The listing builds one solid part. Answer for the finished solid, in the listing's coordinates (mm). Give positions to 0.01 mm unless a question says otherwise; leave off trailing zeros. Order: outer loops, then holes, each group sorted by start corner. A loop starts at its lowest first (then second) coordinate and runs counter-clockwise, first axis right, second up. Notation, with made-up numbers: (-5, -39) - (14, -39) arc R16 ccw to (14, -34) - close; hole circle Ø6 at (-11, 81.5). An arc over 180 degrees is marked (long way). Answer in a Markdown table with one row per item. Add a question column.
```python
from build123d import *

# Parameters (mm, degrees)
F0_W          = 70
F0_H          = 70
F0_W_2        = 1860
F0_H_2        = 360
F1_DEPTH      = 70
F2_W          = 360
F2_H          = 30
F3_DEPTH      = 25
F3_DEPTH_BACK = 25
F4_SCALE      = 0.4


with BuildPart() as f1:
    # F0 (on Front) → F1 (new body)
    with BuildSketch(Plane.XZ):
        with Locations((35, -35)):
            Rectangle(F0_W, F0_H)
        with Locations((1000, -35)):
            Rectangle(F0_W_2, F0_H)
        with Locations((35, -250)):
            Rectangle(F0_W, F0_H_2)
        with Locations((1965, -35)):
            Rectangle(F0_W, F0_H)
        with Locations((35, -465)):
            Rectangle(F0_W, F0_H)
        with Locations((1965, -250)):
            Rectangle(F0_W, F0_H_2)
        with Locations((1000, -465)):
            Rectangle(F0_W_2, F0_H)
        with Locations((1965, -465)):
            Rectangle(F0_W, F0_H)
    extrude(amount=F1_DEPTH)

    # F2 (on face) → F3 (cut, two sides)
    with BuildSketch(Plane.XY) as f3_sk:
        with Locations((1620, -35)):
            Rectangle(F2_W, F2_H)
    extrude(amount=F3_DEPTH, mode=Mode.SUBTRACT)
    extrude(f3_sk.sketch, amount=-F3_DEPTH_BACK, mode=Mode.SUBTRACT)


with BuildPart() as f1_1:
    # F4: moved
    add(f1.part.scale(F4_SCALE).moved(Location((1200, -42, -300))))


solid = f1_1.part
```
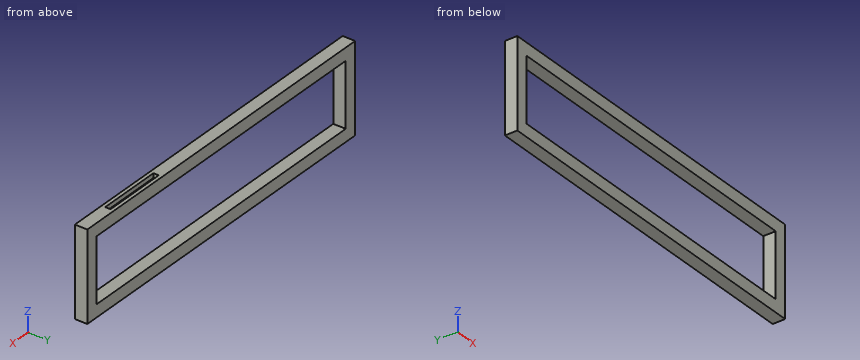
(1) Straight lines are drawn through the part: line 1 (X direction, y = -60.5, z = -379); line 2 (Z direction, x = 1728, y = -53). For each, find the intervals that lie inside material, in ascending order.
(2) Find section A-A, the plane z = -388. Write down the section's boundary in (x, y).
(3) Find section B-B, the plane x = 1843.5. Write down the section's boundary in (y, z).
(4) Find section C-C, the plane x = 1632. Write down the section's boundary in (y, z).
Answer key:
| question | item | result |
|---|---|---|
| 1 | line 1 | 1200 to 1228, 1972 to 2000 |
| 1 | line 2 | -500 to -472, -328 to -300 |
| 2 | outline | (1200, -70) - (1228, -70) - (1228, -42) - (1200, -42) - close; (1972, -70) - (2000, -70) - (2000, -42) - (1972, -42) - close |
| 3 | outline | (-70, -500) - (-42, -500) - (-42, -472) - (-70, -472) - close; (-70, -328) - (-42, -328) - (-42, -300) - (-50, -300) - (-50, -310) - (-62, -310) - (-62, -300) - (-70, -300) - close |
| 4 | outline | (-70, -500) - (-42, -500) - (-42, -472) - (-70, -472) - close; (-70, -328) - (-42, -328) - (-42, -300) - (-70, -300) - close |
